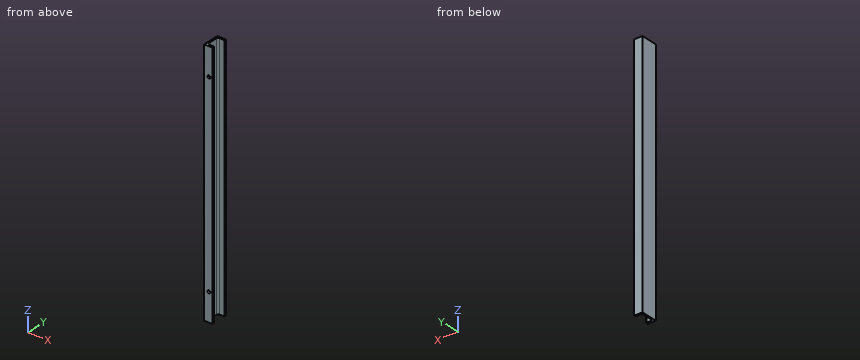
from build123d import *

# Parameters (mm, degrees)
BOSS_EXTRUDE1_DEPTH = 450
SKETCH2_R           = 5.5
CUT_EXTRUDE1_DEPTH  = 10


with BuildPart() as part:
    # Sketch1 → Boss-Extrude1 (new, symmetric)
    with BuildSketch(Plane.XY):
        with BuildLine():
            Line((12, 24), (-3, 24))
            ThreePointArc((-3, 24), (-7.242640687, 22.242640687), (-9, 18))
            Line((-9, 18), (-9, -16))
            ThreePointArc((-9, -16), (-7.242640687, -20.242640687), (-3, -22))
            Line((-3, -22), (12, -22))
            ThreePointArc((12, -22), (14.121320344, -22.878679656), (15, -25))
            Line((15, -25), (15, -30))
            Line((15, -30), (-15, -30))
            Line((-15, -30), (-15, 30))
            Line((-15, 30), (15, 30))
            Line((15, 30), (15, 27))
            ThreePointArc((15, 27), (14.121320344, 24.878679656), (12, 24))
        make_face()
    extrude(amount=BOSS_EXTRUDE1_DEPTH, both=True)

    # Sketch2 → Cut-Extrude1 (cut)
    with BuildSketch(Plane(origin=(0, -22, 0), x_dir=(1, 0, 0), z_dir=(0, 1, 0))):
        with Locations(Location((2, -350, 0), (0, 0, 204.619977329))):
            Circle(SKETCH2_R)
    cut_extrude1 = extrude(amount=-CUT_EXTRUDE1_DEPTH, mode=Mode.SUBTRACT)

    # Mirror1: Cut-Extrude1 across plane
    add(cut_extrude1.mirror(Plane.XY), mode=Mode.SUBTRACT)


solid = part.part
Source: CAD feature listing. Evaluate the final solid. Frame: model axes, mm. Round coordinates to 2 decimals unless told otherwise and drop trailing zeros. Loops run counter-clockwise (first coordinate to the right, second up) from the corner with the lowest first, then second, coordinate; pieces in that order, holes last.
Q1. Ray query, line 1 (Z direction, x = 2, y = -26.25); line 2 (X direction, y = -26.75, z = -350); line 3 (Y direction, x = 7.5, z = 406.5). Return the intervals inside material, ascending.
Q2. Section A-A, the plane x = 2. Return loops of the section in (y, z).
Q3. Section C-C, the plane y = 6. Return loops of the section in (x, z), plus the area to 3 significant figures.
Q4. Section B-B, the plane z = 178.5. Return loops of the section in (x, y), plus the area to 3 significant figures.
Q5. First-contact query: P1, Ø10, axis at y = -3.5, z = -106.5, coming from the +X side; P2, Ø10, axis at y = 14.5, z = 94.5, coming from the +X side; P3, Ø5, axis at y = 20, z = 329.5, coming from the +X side. Flat tips, straight axial feed; report the tip coordinate or a pass-through.
Solutions:
1. line 1: z = -450 to -355.5, -344.5 to 344.5, 355.5 to 450
1. line 2: x = -15 to -3.5, 7.5 to 15
1. line 3: y = -30 to -22, 24 to 30
2. outline: (-30, -450) - (-22, -450) - (-22, -355.5) - (-30, -355.5) - close; (-30, -344.5) - (-22, -344.5) - (-22, 344.5) - (-30, 344.5) - close; (-30, 355.5) - (-22, 355.5) - (-22, 450) - (-30, 450) - close; (24, -450) - (30, -450) - (30, 450) - (24, 450) - close
3. outline: (-15, -450) - (-9, -450) - (-9, 450) - (-15, 450) - close
3. area: 5,400 mm2
4. outline: (-15, -30) - (15, -30) - (15, -25) arc R3 ccw to (12, -22) - (-3, -22) arc R6 cw to (-9, -16) - (-9, 18) arc R6 cw to (-3, 24) - (12, 24) arc R3 ccw to (15, 27) - (15, 30) - (-15, 30) - close
4. area: 708 mm2
5. P1: stops at x = -9
5. P2: stops at x = -8.81
5. P3: stops at x = -6.97
